Autodesk Inventor part; units mm, degrees
ref_plane "Work Plane2" through (-14.7431, -7.9324, 300) normal (0, 0, -1) x (0, 1, 0)
ref_plane "YZ Plane" through (0, 0, 0) normal (1, 0, 0) x (0, 1, 0)
ref_plane "XZ Plane" through (0, 0, 0) normal (0, 1, 0) x (-1, 0, 0)
ref_plane "Work Plane1" through (0, 0, 0) normal (0, 0, 1) x (1, 0, 0)
sketch "Sketch1" plane through (0, 0, 0) normal (0, 0, 1) x (1, 0, 0)
  circle A0 centre (-0.378, 7.3806) radius 0.75
  line L0 (-0.756, 75) -> (0, 75) construction
  arc A1 (-13.4366, 0) -> (12.6806, 0) centre (-0.378, 7.3806) ccw construction
  arc A2 (-12.1028, 9.8588) -> (11.3464, 9.8606) centre (-0.378, 7.3806) ccw
  line L1 (-12.3298, 8.256) -> (-11.557, 13.7119)
  line L2 (11.5739, 8.2546) -> (10.8008, 13.7119)
  line L3 (-12.3298, 8.256) -> (-0.756, 75)
  line L4 (-0.756, 75) -> (0, 75)
  line L5 (0, 75) -> (11.5739, 8.2546)
  spline S0 degree 3 poles (0, 75) (0.0654, 74.6898) (0.2183, 73.9622) (0.6185, 72.0374) (0.8255, 71.0325) (1.5395, 67.5353) (2.0401, 65.0263) (3.7365, 56.3358) (4.8865, 50.1031) (8.482, 29.574) (10.8053, 14.5022) (12.6806, 0) knots -7.652768 -7.652768 -7.652768 -7.652768 -7.375677 -7.375677 -7.074889 -7.074889 -6.315253 -6.315253 -4.432937 -4.432937 -0.050389 -0.050389 -0.050389 -0.050389
  spline S1 degree 3 poles (-13.4366, 0) (-10.3976, 23.501) (-6.0464, 49.5688) (-0.9743, 73.9622) (-0.8214, 74.6898) (-0.756, 75) knots -2.513741 -2.513741 -2.513741 -2.513741 -0.095109 -0.095109 0 0 0 0
  point P0 (0, 0)
ref_plane "Work Plane2" through (-14.7431, -7.9324, 300) normal (0, 0, -1) x (0, 1, 0)
extrude "Extrusion1" add sketch "Sketch1" along normal up to surface (300 mm away) contours L3 L4 L5 A2
properties part number "Vtail"
Input: part model. Units: mm. Frame: model coordinates. Give positions to 0.01 mm unless a question says otherwise; leave off trailing zeros. Order: outer loops, then holes, each group sorted by start corner. A loop starts at its lowest first (then second) coordinate and runs counter-clockwise, first axis right, second up. Notation, with made-up numbers: (29, -21) - (78, -21) arc R15 cw to (78, -15) - close; hole circle Ø9 at (34, -24.5). An arc over 180 degrees is marked (long way). Use a Markdown table: item, result.
(1) Section query C-C (x = 4). Output: boundary loops of the cut face in (y, z).
Computed values:
| item | result |
|---|---|
| outline | (-3.77, 0) - (51.93, 0) - (51.93, 300) - (-3.77, 300) - close |
(2) Section query B-B (y = 61.5). Output: boundary loops of the cut face in (x, z), then the cut area to 3 significant figures.
Computed values:
| item | result |
|---|---|
| outline | (-3.1, 0) - (2.34, 0) - (2.34, 300) - (-3.1, 300) - close |
| area | 1,630 mm2 |
(3) Pin query (flat end, axial travel): pin 1 (3 mm diameter, centred on y = 5.5, z = 185, fed in from +X); pin 2 (2 mm diameter, centred on y = 43, z = 130, fed in from -X); pin 3 (5 mm diameter, centred on y = 59, z = 201, fed in from +X). Return the tip coordinate at first contact, or that it passes through.
Computed values:
| item | result |
|---|---|
| pin 1 | stops at x = 11.6 |
| pin 2 | stops at x = -6.48 |
| pin 3 | stops at x = 3.21 |
(4) Line query: line 1 (Y direction, x = -0.5, z = 103.5); line 2 (X direction, y = -1, z = 197); line 3 (X direction, y = 68, z = 111.5). Output: solid intervals per line, ascending. Write a range as from..to.
Computed values:
| item | result |
|---|---|
| line 1 | y = -4.6..6.64, 8.12..75 |
| line 2 | x = -8.94..8.19 |
| line 3 | x = -1.97..1.21 |
(5) Section query A-A (z = 101). Output: boundary loops of the cut face in (x, y).
Computed values:
| item | result |
|---|---|
| outline | (-12.33, 8.26) arc R11.98 ccw (long way) to (11.57, 8.25) - (0, 75) - (-0.76, 75) - close; hole circle Ø1.5 at (-0.38, 7.38) |
